Part model, mm, in its own coordinate system. A direction names the side the tool comes from. Coordinates: 2 decimals unless noted, no trailing zeros. Write each loop counter-clockwise with the first axis right and the second up, starting at its lowest first coordinate (ties: lowest second). Pieces come first, ordered by that corner, then holes. Notation, with made-up numbers: (38, 44.5) - (74, 44.5) arc R10 cw to (74, 50.5) - close; hole circle Ø6 at (37, -37.75). An arc over 180 degrees is marked (long way). Use a Markdown table: item, result.
```python
from build123d import *

# Parameters (mm, degrees)
F0_W          = 70
F0_H          = 140
F1_DEPTH      = 7
F2_R          = 5
F3_T          = -2.5
F4_W          = 105
F4_H          = 14
F4_R          = 2.5
F5_DEPTH      = 2
F7_DEPTH      = 2
F7_DEPTH_BACK = 2


with BuildPart() as f1:
    # F0 (on Front) → F1 (new body)
    with BuildSketch(Plane.XZ):
        Rectangle(F0_W, F0_H)
    extrude(amount=F1_DEPTH)

    # F2
    f2_edges = [f1.edges().sort_by_distance(p)[0] for p in [
        (35, -3.5, 70),
        (35, -3.5, -70),
        (-35, -3.5, -70),
        (-35, -3.5, 70),
    ]]
    fillet(f2_edges, radius=F2_R)

    # F3
    f3_openings = [f1.faces().sort_by_distance(p)[0] for p in [
        (0, -7, 0),
    ]]
    offset(amount=F3_T, openings=f3_openings)

    # F4 (on face) → F5 (join)
    with BuildSketch(Plane(origin=(0, 0, 0), x_dir=(-1, 0, 0), z_dir=(0, 1, 0))):
        with Locations((-87.5, 0)):
            Rectangle(F4_W, F4_H)
        with BuildLine():
            Line((-35, -7), (0, -7))
            ThreePointArc((0, -7), (7, 0), (0, 7))
            Line((0, 7), (-35, 7))
            Line((-35, 7), (-35, -7))
        make_face()
        Circle(F4_R, mode=Mode.SUBTRACT)
    extrude(amount=F5_DEPTH)

    # F6 (on face) → F7 (join, two sides)
    with BuildSketch(Plane.XZ) as f7_sk:
        Polygon((160, 27), (140, 7), (140, -7), (160, -27), align=None)
    extrude(amount=-F7_DEPTH)
    extrude(f7_sk.sketch, amount=F7_DEPTH_BACK)


solid = f1.part
```
Item 1: Drill centre lines: probe 1 along X at (y, z) = (-3.5, 2.5); probe 2 along Z at (x, y) = (18.5, -4); probe 3 along X at (y, z) = (-0.25, 4). Where is each one in solid material? Low to high.
From the geometry:
| item | result |
|---|---|
| probe 1 | -35 to -32.5, 32.5 to 35 |
| probe 2 | -70 to -67.5, 67.5 to 70 |
| probe 3 | -35 to 35, 140 to 160 |
Item 2: Band-saw the part on B-B, the plane y = -4.25. Give the cut face in (x, z).
From the geometry:
| item | result |
|---|---|
| outline | (-35, -65) arc R5 ccw to (-30, -70) - (30, -70) arc R5 ccw to (35, -65) - (35, 65) arc R5 ccw to (30, 70) - (-30, 70) arc R5 ccw to (-35, 65) - close; hole (-32.5, -65) arc R2.5 ccw to (-30, -67.5) - (30, -67.5) arc R2.5 ccw to (32.5, -65) - (32.5, 65) arc R2.5 ccw to (30, 67.5) - (-30, 67.5) arc R2.5 ccw to (-32.5, 65) - close |
Item 3: Band-saw the part on A-A, the plane z = 56. Give the cut face in (x, y).
From the geometry:
| item | result |
|---|---|
| outline | (-35, -7) - (-32.5, -7) - (-32.5, -2.5) - (32.5, -2.5) - (32.5, -7) - (35, -7) - (35, 0) - (-35, 0) - close |
Item 4: Which spindle directions (+Z, -Z, +X, -X, +Y, -Y) get a long thin tool onto all of the face, cutting with end or side? Do faces 5 (the face through (32.5, -5, -1)), 6 (the face through (0.54, 0.99, -2.44)), 7 (the face through (150, 0, 17)), 8 (the face through (152, -2, 0)). Say none if no direction does.
From the geometry:
| item | result |
|---|---|
| face 5 | -Y |
| face 6 | +Y |
| face 7 | +Z, +Y, -Y |
| face 8 | +Z, -Z, +X, -Y |
Item 5: Two-plate mould, pull along X, no slides. Class faces 1 (the face through (-7, 1, 0)), 2 (the face through (0, -5, -67.5)), 3 (the face through (33, -4, -69)), 4 (the face through (-8, 0, 1)): pulls with the +X half, pulls with the -X half, needs draft (parallel to the pull), parting line crosses it, or undercut.
From the geometry:
| item | result |
|---|---|
| face 1 | pulls with the -X half |
| face 2 | undercut |
| face 3 | pulls with the +X half |
| face 4 | needs draft |
Item 6: Drop flat-ended pins along their axis: P1, Ø1.6, axis at x = 93, y = 1, coming from the +Z side; P2, Ø3, axis at x = -3, z = -29.5, coming from the -Y side; P3, Ø1.5, axis at y = -6, z = -11.5, coming from the +X side. Give the stop position or say it passes through.
From the geometry:
| item | result |
|---|---|
| P1 | z = 7 |
| P2 | y = -2.5 |
| P3 | x = 35 |
Item 7: Band-saw the part on C-C, the plane x = 8. Give the cut face in (y, z).
From the geometry:
| item | result |
|---|---|
| outline | (-7, -70) - (0, -70) - (0, -7) - (2, -7) - (2, 7) - (0, 7) - (0, 70) - (-7, 70) - (-7, 67.5) - (-2.5, 67.5) - (-2.5, -67.5) - (-7, -67.5) - close |
Item 8: Band-saw the part on D-D, the plane z = 0. Give the cut face in (x, y).
From the geometry:
| item | result |
|---|---|
| outline | (-35, -7) - (-32.5, -7) - (-32.5, -2.5) - (32.5, -2.5) - (32.5, -7) - (35, -7) - (35, 0) - (140, 0) - (140, -2) - (160, -2) - (160, 2) - (2.5, 2) - (2.5, 0) - (-2.5, 0) - (-2.5, 2) - (-7, 2) - (-7, 0) - (-35, 0) - close |
